Part model, mm, in its own coordinate system. Face numbers are marked on the shaded views. A direction names the side the tool comes from. Round coordinates to 2 decimals unless told otherwise and drop trailing zeros. Write each loop counter-clockwise with the first axis right and the second up, starting at its lowest first coordinate (ties: lowest second). Pieces come first, ordered by that corner, then holes. Notation, with made-up numbers: M 12.5,-3.5 L 38.5,-3.5 A8 ccw 38.5,5.5 Z; hole C 49.25,-37.5 d1. An arc over 180 degrees is marked long. Use one line per item in the form item = value. Start each with the question number.
Item 1: Flat gauge pins, fed straight in: pin 1 Ø14.5 at (x, y) = (9.5, -13.5) entering from +Z; pin 2 Ø6 at (x, z) = (-5.5, 44.5) entering from -Y; pin 3 Ø2 at (x, y) = (24, -3) entering from +Z. Where does each tip first touch, or does it go through?
Item 2: Which spindle directions (+Z, -Z, +X, -X, +Y, -Y) get a long thin tool onto all of the face, cutting with end or side? Do the marked faces 4, 5 and 6. Say none if no direction does.
Item 3: Cut at D-D, the plane z = 50. Give the cut face in (x, y).
Item 4: Cut at C-C, the plane x = 25.5. Give the cut face in (y, z).
Item 5: Mould opens along X. For the marked faces 1, 2 and 3 say: +X half, -X half, draft (parallel to the pull), parting line (faces both ways), or undercut.
Item 6: Cut at A-A, the plane z = 32.5. Give the cut face in (x, y), then the cut area to 3 significant figures.
Item 7: Probe L1, parallel to X at y = -21.5, z = 21.5; L2, parallel to X at y = -13.75, z = 57.5; L3, parallel to Z at x = -9, y = -22. List the from-to ranges inside material, lowest first.
Item 8: Cut at B-B, the plane y = -23. Give the cut face in (x, z), then the cut area to 3 significant figures.
from build123d import *

# Parameters (mm, degrees)
F1_DEPTH  = 30
F1_FACE_W = 15
F1_FACE_H = 30
F2_DEPTH  = 25


with BuildPart() as f1:
    # F0 (on Front) → F1 (new body)
    with BuildSketch(Plane.XZ):
        Polygon((-25.400001, 0), (33.599999, 0), (33.599999, 35), (18.599999, 35), (18.599999, 15), (-10.400001, 15), (-10.400001, 35), (-25.400001, 35), align=None)
    extrude(amount=F1_DEPTH)

    # F1_face (on face) → F2 (join)
    with BuildSketch(Plane(origin=(-17.900001, -15, 35), x_dir=(1, 0, 0), z_dir=(0, 0, 1))):
        Rectangle(F1_FACE_W, F1_FACE_H)
    extrude(amount=F2_DEPTH)


solid = f1.part
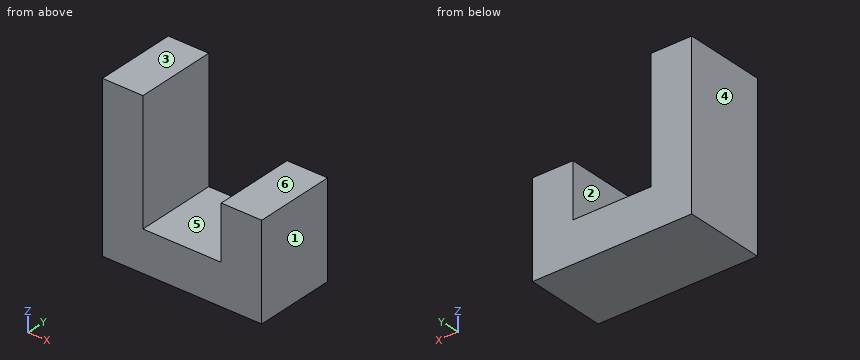
Model answer:
q1.pin_1 = 15
q1.pin_2 = through
q1.pin_3 = 35
q2.face_4 = +Z, -Z, -X, +Y, -Y
q2.face_5 = +Z, +Y, -Y
q2.face_6 = +Z, +X, +Y, -Y
q3.outline = M -25.4,-30 L -10.4,-30 L -10.4,0 L -25.4,0 Z
q4.outline = M -30,0 L 0,0 L 0,35 L -30,35 Z
q5.face_1 = +X half
q5.face_2 = undercut
q5.face_3 = draft
q6.outline = M -25.4,-30 L -10.4,-30 L -10.4,0 L -25.4,0 Z; M 18.6,-30 L 33.6,-30 L 33.6,0 L 18.6,0 Z
q6.area = 900 mm²
q7.L1 = -25.4 to -10.4, 18.6 to 33.6
q7.L2 = -25.4 to -10.4
q7.L3 = 0 to 15
q8.outline = M -25.4,0 L 33.6,0 L 33.6,35 L 18.6,35 L 18.6,15 L -10.4,15 L -10.4,60 L -25.4,60 Z
q8.area = 1,860 mm²
